For this review, take the finished solid that the model builds, in its own axes (mm). A direction names the side the tool comes from. Round coordinates to 2 decimals unless told otherwise and drop trailing zeros. Loops run counter-clockwise (first coordinate to the right, second up) from the corner with the lowest first, then second, coordinate; pieces in that order, holes last. Notation, with made-up numbers: M 83,54 L 140,54 A30 cw 140,88 Z; hole C 34,-4.75 d4. An arc over 180 degrees is marked long. One line per question, with ' | ' between items. Start each with the question number.
1) For faces 1 (the face through (863.6, 19, 89)), 2 (the face through (613, 19, 179.388)), 3 (the face through (774.7, 19, 19)), 4 (the face through (770, 19, 141.275)), 5 (the face through (487.362, 19, 132)), list the 3-axis set-ups (+Z, -Z, +X, -X, +Y, -Y) from which the entire face can be reached by the end or side of a thin tool; tool diameter is ignored.
2) We need section D-D (x = 809.5). Give the boundary of the cut face in (y, z), and give its area (3 significant figures).
3) For pin 1 Ø19 at (y, z) = (14.5, 17) entering from +X; pin 2 Ø19 at (y, z) = (22.5, 157.5) entering from +X, all flat-tipped, find the tip position at first contact; note any pin that passes through.
4) We need section B-B (y = 27). Give the boundary of the cut face in (x, z).
5) We need section A-A (z = 149). Give the boundary of the cut face in (x, y), and give its area (3 significant figures).
6) Mouldability with a two-part tool opening along Z and no side actions: class faces 6 (the face through (544.512, 19, 150)), 7 (the face through (645.3, 18.8, 68.2)), 8 (the face through (471, 19, 141.288)) as pulls with the +Z half, pulls with the -Z half, needs draft (parallel to the pull), parting line crosses it, or undercut.
7) For probe 1 along X at (y, z) = (14.5, 125.5); probe 2 along Z at (x, y) = (536.5, 4); probe 3 along Z at (x, y) = (704.5, 20), list the stretches that pass through material, from the lowest coordinate up. Write a range as from..to.
8) We need section C-C (x = 463). Give the boundary of the cut face in (y, z).
```python
from build123d import *

# Parameters (mm, degrees)
SKETCH1_R           = 19.05
BOSS_EXTRUDE1_DEPTH = 38.1
CUT_EXTRUDE5_DEPTH  = 39.1
SKETCH8_W           = 184.15
SKETCH8_H           = 38.1127
CUT_EXTRUDE6_DEPTH  = 39.1


with BuildPart() as part:
    # Sketch1 → Boss-Extrude1 (new body)
    with BuildSketch(Plane(origin=(0, 0, 0), x_dir=(1, 0, 0), z_dir=(0, 1, 0))):
        Polygon((0, 0), (774.7, 0), (774.7, -38.1), (863.6, -38.1), (863.6, -179.3875), (0, -179.3875), align=None)
        with Locations((627.126, -73.914)):
            Circle(SKETCH1_R, mode=Mode.SUBTRACT)
    extrude(amount=BOSS_EXTRUDE1_DEPTH)

    # Sketch7 → Cut-Extrude5 (cut, through all)
    with BuildSketch(Plane(origin=(0, 38.1, 0), x_dir=(1, 0, 0), z_dir=(0, 1, 0))):
        Polygon((455.6125, -141.2875), (487.3625, -141.2875), (487.3625, -122.2375), (544.5125, -122.2375), (544.5125, -179.3875), (455.6125, -179.3875), align=None)
    extrude(amount=-CUT_EXTRUDE5_DEPTH, mode=Mode.SUBTRACT)

    # Sketch8 → Cut-Extrude6 (cut, through all)
    with BuildSketch(Plane(origin=(0, 38.1, 0), x_dir=(1, 0, 0), z_dir=(0, 1, 0))):
        with Locations((771.525, -160.33115)):
            Rectangle(SKETCH8_W, SKETCH8_H)
    extrude(amount=-CUT_EXTRUDE6_DEPTH, mode=Mode.SUBTRACT)


solid = part.part
```
Answers below:
1) face 1: +Z, -Z, +X, +Y, -Y | face 2: +Z, +X, -X, +Y, -Y | face 3: -Z, +X, +Y, -Y | face 4: +Z, +X, +Y, -Y | face 5: +Z, +Y, -Y
2) outline: M 0,38.1 L 38.1,38.1 L 38.1,141.27 L 0,141.27 Z | area: 3,930 mm^2
3) pin 1: x = 774.7 | pin 2: x = 679.45
4) outline: M 0,0 L 774.7,0 L 774.7,38.1 L 863.6,38.1 L 863.6,141.27 L 679.45,141.27 L 679.45,179.39 L 544.51,179.39 L 544.51,122.24 L 487.36,122.24 L 487.36,141.29 L 455.61,141.29 L 455.61,179.39 L 0,179.39 Z; hole C 627.13,73.91 d38.1
5) outline: M 0,0 L 455.61,0 L 455.61,38.1 L 0,38.1 Z; M 544.51,0 L 679.45,0 L 679.45,38.1 L 544.51,38.1 Z | area: 22,500 mm^2
6) face 6: needs draft | face 7: undercut | face 8: pulls with the +Z half
7) probe 1: 0..487.36, 544.51..863.6 | probe 2: 0..122.24 | probe 3: 0..141.27
8) outline: M 0,0 L 38.1,0 L 38.1,141.29 L 0,141.29 Z
